```python
from build123d import *

# Parameters (mm, degrees)
SKETCH1_R           = 10
SKETCH1_R_2         = 5
BOSS_EXTRUDE1_DEPTH = 30
FILLET1_R           = 3
SKETCH5_R           = 30
SKETCH5_R_2         = 25
BOSS_EXTRUDE2_DEPTH = 5
FILLET2_R           = 1


with BuildPart() as part:
    # Sketch1 → Boss-Extrude1 (new body)
    with BuildSketch(Plane.XY):
        Circle(SKETCH1_R)
        Circle(SKETCH1_R_2, mode=Mode.SUBTRACT)
    extrude(amount=BOSS_EXTRUDE1_DEPTH)

    # Sketch4 → Revolve1 (revolve)
    with BuildSketch(Plane(origin=(0, 0, 0), x_dir=(1, 0, 0), z_dir=(0, 1, 0))):
        Polygon((10, -5), (30, -5), (30, -7), (25, -9.886751346), (25, -20.113248654), (30, -23), (30, -25), (10, -25), align=None)
    revolve(axis=Axis((0, 0, 0), (0, 0, 1)))

    # Fillet1
    fillet1_edges = [part.edges().sort_by_distance(p)[0] for p in [
        (-25, 0, 20.113248654),
        (-25, 0, 9.886751346),
    ]]
    fillet(fillet1_edges, radius=FILLET1_R)

    # Sketch5 → Boss-Extrude2 (add)
    with BuildSketch(Plane.XY.offset(18.381197846)):
        Circle(SKETCH5_R)
        Circle(SKETCH5_R_2, mode=Mode.SUBTRACT)
    extrude(amount=-BOSS_EXTRUDE2_DEPTH)

    # Fillet2
    fillet2_edges = [part.edges().sort_by_distance(p)[0] for p in [
        (-30, 0, 13.381197846),
        (-30, 0, 18.381197846),
    ]]
    fillet(fillet2_edges, radius=FILLET2_R)


solid = part.part
```
Input: part model. Units: mm. Frame: model coordinates. A direction names the side the tool comes from. Round coordinates to 2 decimals unless told otherwise and drop trailing zeros. Loops run counter-clockwise (first coordinate to the right, second up) from the corner with the lowest first, then second, coordinate; pieces in that order, holes last. Notation, with made-up numbers: (28.5, 72.5) -> (58.5, 72.5) arc R24 cw to (58.5, 99.5) -> close; hole circle Ø2 at (11, -34.75). An arc over 180 degrees is marked (long way). Write each question's results on one line, items separated by ' | '.
1. First-contact query: P1, Ø12, axis at y = -20.5, z = 4, coming from the -X side; P2, Ø12, axis at x = 11.5, y = -21, coming from the -Z side; P3, Ø5, axis at y = 9.5, z = 25.5, coming from the +X side; P4, Ø16, axis at x = 0, y = 0, coming from the +Z side. Flat tips, straight axial feed; report the tip coordinate or a pass-through.
Geometry results:
P1: x = -26.22 | P2: z = 5 | P3: x = 29.16 | P4: z = 30
2. Mould query, pull axis X, two halves, no side actions, for faces 1 (the face through (-1.08, -4.88, 14.79)), 2 (the face through (-29.97, 1.32, 6.01)), 3 (the face through (13, 22, 13.381)). Classes: +X half, -X half, draft (parallel to the pull), parting line (faces both ways), or undercut.
Geometry results:
face 1: undercut | face 2: parting line | face 3: draft
3. Ray query, line 1 (Z direction, x = -15, y = 25); line 2 (Y direction, x = 0, z = 24); line 3 (Y direction, x = 0, z = 11.75). Return the intervals inside material, ascending. Write a range as from..to.
Geometry results:
line 1: 5..7.49, 13.39..18.37, 22.51..25 | line 2: -30..-5, 5..30 | line 3: -25..-5, 5..25
4. Section A-A (z = 6). Return loops of the section in (x, y).
Geometry results:
outline: circle Ø60 at (0, 0); hole circle Ø10 at (0, 0)
5. Section B-B (z = 22.25). Return loops of the section in (x, y).
Geometry results:
outline: circle Ø57.4 at (0, 0); hole circle Ø10 at (0, 0)
6. Set-up query: faces 4 (the face through (23.846, 7.509, 12.512)), 5 (the face through (-2.17, -9.76, 27.46)), 6 (the face through (-13, 0, 5)), 7 (the face through (-5, -2, 30)). Return all of +Z, -Z, +X, -X, +Y, -Y with unobstructed straight access to the full face (end or side cutting, diameter ignored); none if empty.
Geometry results:
face 4: none | face 5: +Z | face 6: -Z | face 7: +Z, +X, -X, +Y, -Y
